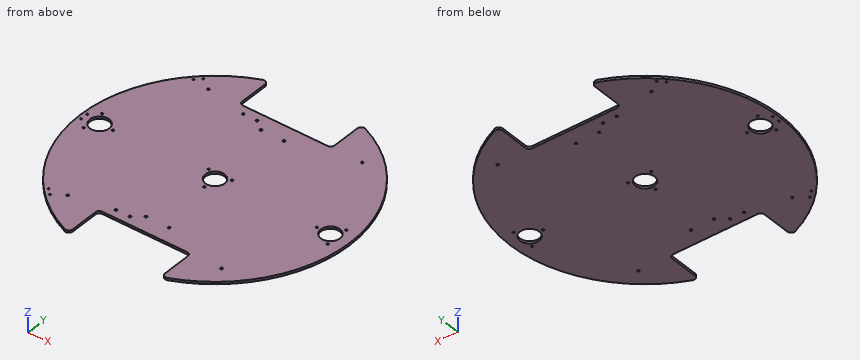
from build123d import *

# Parameters (mm, degrees)
SKETCH_1_R           = 175
EXTRUDE_1_DEPTH      = 3
CUT_EXTRUDE_1_DEPTH  = 3
FILLET_1_R           = 5
FILLET_2_R           = 5
FILLET_3_R           = 5
SKETCH_5_R           = 1.5
CUT_EXTRUDE_4_DEPTH  = 3
SKETCH_10_R          = 12.5
SKETCH_10_R_2        = 1.3
CUT_EXTRUDE_13_DEPTH = 10
SKETCH_14_R          = 1.1
CUT_EXTRUDE_14_DEPTH = 10
SKETCH_12_R          = 1.5
CUT_EXTRUDE_17_DEPTH = 10
SKETCH_13_R          = 1.5
CUT_EXTRUDE_18_DEPTH = 5


with BuildPart() as part:
    # ｽｹｯﾁ1 → ﾎﾞｽ - 押し出し1 (new body)
    with BuildSketch(Plane.XY):
        Circle(SKETCH_1_R)
    extrude(amount=EXTRUDE_1_DEPTH)

    # ｽｹｯﾁ2 → ｶｯﾄ - 押し出し1 (cut)
    with BuildSketch(Plane.XY.offset(3)):
        with BuildLine():
            Line((-60, 115), (0, 115))
            Line((0, 115), (0, 175))
            ThreePointArc((0, 175), (-30.465194158, 172.327803749), (-60, 164.392822228))
            Line((-60, 164.392822228), (-60, 115))
        make_face()
        with BuildLine():
            Line((0, 175), (0, 115))
            Line((0, 115), (60, 115))
            Line((60, 115), (60, 164.392822228))
            ThreePointArc((60, 164.392822228), (30.465194158, 172.327803749), (0, 175))
        make_face()
        with BuildLine():
            Line((0, -175), (0, -115))
            Line((0, -115), (-60, -115))
            Line((-60, -115), (-60, -164.392822228))
            ThreePointArc((-60, -164.392822228), (-30.465194158, -172.327803749), (0, -175))
        make_face()
        with BuildLine():
            Line((60, -115), (0, -115))
            Line((0, -115), (0, -175))
            ThreePointArc((0, -175), (30.465194158, -172.327803749), (60, -164.392822228))
            Line((60, -164.392822228), (60, -115))
        make_face()
    extrude(amount=-CUT_EXTRUDE_1_DEPTH, mode=Mode.SUBTRACT)

    # ﾌｨﾚｯﾄ1
    fillet_1_edges = [part.edges().sort_by_distance(p)[0] for p in [
        (-60, 164.392822228, 1.5),
    ]]
    fillet(fillet_1_edges, radius=FILLET_1_R)

    # ﾌｨﾚｯﾄ2
    fillet_2_edges = [part.edges().sort_by_distance(p)[0] for p in [
        (-60, 115, 1.5),
        (60, 164.392822228, 1.5),
        (60, 115, 1.5),
    ]]
    fillet(fillet_2_edges, radius=FILLET_2_R)

    # ﾌｨﾚｯﾄ3
    fillet_3_edges = [part.edges().sort_by_distance(p)[0] for p in [
        (-60, -115, 1.5),
        (60, -115, 1.5),
        (60, -164.392822228, 1.5),
        (-60, -164.392822228, 1.5),
    ]]
    fillet(fillet_3_edges, radius=FILLET_3_R)

    # ｽｹｯﾁ5 → ｶｯﾄ - 押し出し4 (cut)
    with BuildSketch(Plane.XY.offset(3)):
        with Locations((-100, -115)):
            Circle(SKETCH_5_R)
        with Locations((100, -115)):
            Circle(SKETCH_5_R)
        with Locations((100, 115)):
            Circle(SKETCH_5_R)
        with Locations((-100, 115)):
            Circle(SKETCH_5_R)
    extrude(amount=-CUT_EXTRUDE_4_DEPTH, mode=Mode.SUBTRACT)

    # ｽｹｯﾁ10 → ｶｯﾄ - 押し出し13 (cut)
    with BuildSketch(Plane.XY.offset(3)):
        with Locations((-150, 0)):
            Circle(SKETCH_10_R)
        with Locations((150, 0)):
            Circle(SKETCH_10_R)
        Circle(SKETCH_10_R)
        with Locations((132.5, 0)):
            Circle(SKETCH_10_R_2)
        with Locations((158.75, 15.155444566)):
            Circle(SKETCH_10_R_2)
        with Locations((158.75, -15.155444566)):
            Circle(SKETCH_10_R_2)
        with Locations((-15.155444566, 8.75)):
            Circle(SKETCH_10_R_2)
        with Locations((15.155444566, 8.75)):
            Circle(SKETCH_10_R_2)
        with Locations((0, -17.5)):
            Circle(SKETCH_10_R_2)
        with Locations((-158.75, 15.155444566)):
            Circle(SKETCH_10_R_2)
        with Locations((-158.75, -15.155444566)):
            Circle(SKETCH_10_R_2)
        with Locations((-132.632898389, 0)):
            Circle(SKETCH_10_R_2)
    extrude(amount=-CUT_EXTRUDE_13_DEPTH, mode=Mode.SUBTRACT)

    # ｽｹｯﾁ14 → ｶｯﾄ - 押し出し14 (cut)
    with BuildSketch(Plane.XY.offset(3)):
        with Locations((-170, 5)):
            Circle(SKETCH_14_R)
        with Locations((-170, -5)):
            Circle(SKETCH_14_R)
        with Locations((-114.933514447, 125.360628815)):
            Circle(SKETCH_14_R)
        with Locations((-122.102620524, 118.388977786)):
            Circle(SKETCH_14_R)
        with Locations((-122.102620524, -118.388977786)):
            Circle(SKETCH_14_R)
        with Locations((-114.933514447, -125.360628815)):
            Circle(SKETCH_14_R)
    extrude(amount=-CUT_EXTRUDE_14_DEPTH, mode=Mode.SUBTRACT)

    # ｽｹｯﾁ12 → ｶｯﾄ - 押し出し17 (cut)
    with BuildSketch(Plane.XY.offset(3)):
        with Locations((-15, 94)):
            Circle(SKETCH_12_R)
        with Locations((15, 94)):
            Circle(SKETCH_12_R)
        with Locations((-15, -94)):
            Circle(SKETCH_12_R)
        with Locations((15, -94)):
            Circle(SKETCH_12_R)
    extrude(amount=-CUT_EXTRUDE_17_DEPTH, mode=Mode.SUBTRACT)

    # ｽｹｯﾁ13 → ｶｯﾄ - 押し出し18 (cut)
    with BuildSketch(Plane.XY.offset(3)):
        with Locations((-28, -104)):
            Circle(SKETCH_13_R)
        with Locations((-46, -104)):
            Circle(SKETCH_13_R)
        with Locations((-46, 104)):
            Circle(SKETCH_13_R)
        with Locations((-28, 104)):
            Circle(SKETCH_13_R)
    extrude(amount=-CUT_EXTRUDE_18_DEPTH, mode=Mode.SUBTRACT)


solid = part.part
The listing builds one solid part. Answer for the finished solid, in the listing's coordinates (mm). Coordinates: 2 decimals unless noted, no trailing zeros. Order: outer loops, then holes, each group sorted by start corner. A loop starts at its lowest first (then second) coordinate and runs counter-clockwise, first axis right, second up.
Q1. Given P1, Ø2, axis at x = -15.16, y = 8.75, coming from the +Z side, flat-ended and moving along its own axis, determine where the tip first touches the part or whether it passes through.
Q2. A cutting plane is placed at A-A, the plane x = 143. Write down the section's boundary in (y, z).
Q3. A cutting plane is placed at C-C, the plane y = 75.5. Write down the section's boundary in (x, z).
Q4. Consider line 1 (Y direction, x = 15, z = 2.25); line 2 (Y direction, x = -46, z = 2.2); line 3 (X direction, y = 14, z = 0.9). Determine where each line is inside the solid, lowest interval first.
Q5. A cutting plane is placed at B-B, the plane z = 1.65. State how many separate pieces and enclosed holes the cut face has, and give its area (3 significant figures).
Answers follow:
1. P1: passes through
2. outline: (-100.88, 0) - (-10.36, 0) - (-10.36, 3) - (-100.88, 3) - close; (10.36, 0) - (100.88, 0) - (100.88, 3) - (10.36, 3) - close
3. outline: (-157.88, 0) - (157.88, 0) - (157.88, 3) - (-157.88, 3) - close
4. line 1: y = -115 to -95.5, -92.5 to 7.46, 10.04 to 92.5, 95.5 to 115
4. line 2: y = -115 to -105.5, -102.5 to 102.5, 105.5 to 115
4. line 3: x = -174.44 to -159.35, -158.15 to 158.15, 159.35 to 174.44
5. separate pieces: 1
5. enclosed holes: 30
5. area: 81,000 mm2
